Drawing for the job (mm, zero at the part's lowest x, y, z). Coordinates: 2 decimals unless noted, no trailing zeros. Loops run counter-clockwise (first coordinate to the right, second up) from the corner with the lowest first, then second, coordinate; pieces in that order, holes last.
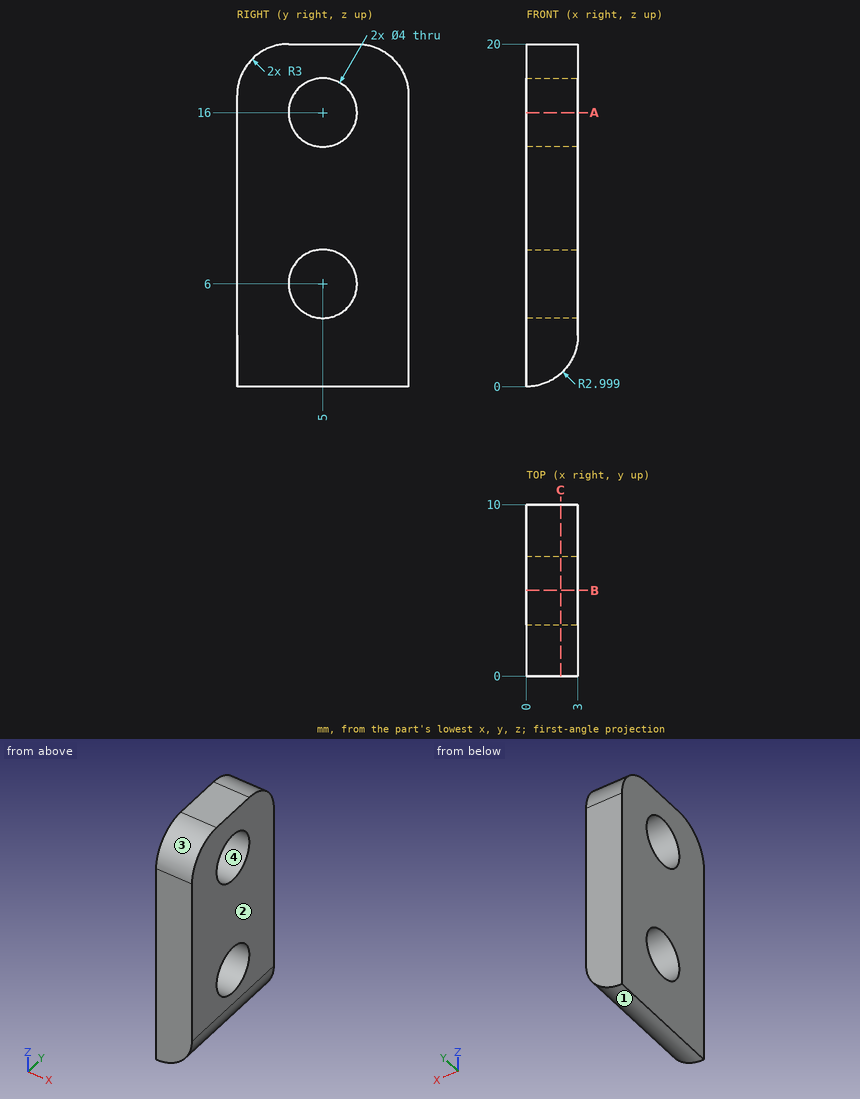
Q1. Probe line 1 (Y direction, x = 2.45, z = 16); line 2 (Y direction, x = 2.65, z = 4.25) (1 decimal); line 3 (Z direction, x = 2.45, y = 6) (1 decimal). List the from-to ranges inside material, lowest first.
Q2. Mould opens along Z. For the marked faces 1, 2, 3 and 4 say: released by +Z, released by -Z, zero draft, split by the parting line, or undercut.
Q3. Saw through at B-B (y = 5). Count the separate pieces of the cut face and the enclosed holes in it.
Q4. Saw through at C-C (x = 2). List the corners of the cut face in (y, z).
Q5. Saw through at A-A (z = 16). List the corners of the cut face in (x, y).
Checked values:
1. line 1: y = 0 to 3, 7 to 10
1. line 2: y = 0 to 4, 6 to 10
1. line 3: z = 1.3 to 4.3, 7.7 to 14.3, 17.7 to 20
2. face 1: released by -Z
2. face 2: zero draft
2. face 3: released by +Z
2. face 4: undercut
3. separate pieces: 3
3. enclosed holes: 0
4. outline: (0, 0.76) - (10, 0.76) - (10, 17) arc R3 ccw to (7, 20) - (3, 20) arc R3 ccw to (0, 17) - close; hole circle Ø4 at (5, 6); hole circle Ø4 at (5, 16)
5. outline: (0, 0) - (3, 0) - (3, 3) - (0, 3) - close; (0, 7) - (3, 7) - (3, 10) - (0, 10) - close
